Design review of the part built by this model. Coordinates are the model's own, in mm. Face numbers are marked on the shaded views. A direction names the side the tool comes from. Give positions to 0.01 mm unless a question says otherwise; leave off trailing zeros. Write each loop counter-clockwise with the first axis right and the second up, starting at its lowest first coordinate (ties: lowest second). Pieces come first, ordered by that corner, then holes. Notation, with made-up numbers: (73.5, 74) -> (101.5, 74) arc R11 cw to (101.5, 86) -> close; hole circle Ø3 at (-25, 31). An arc over 180 degrees is marked (long way). Answer as a JSON object with one key per item and string values.
Autodesk Inventor part; units mm, degrees
ref_plane "YZ Plane" through (0, 0, 0) normal (1, 0, 0) x (0, 1, 0)
ref_plane "XZ Plane" through (0, 0, 0) normal (0, 1, 0) x (-1, 0, 0)
ref_plane "XY Plane" through (0, 0, 0) normal (0, 0, 1) x (1, 0, 0)
sketch "Sketch1" plane through (0, 0, 0) normal (0, 0, 1) x (1, 0, 0)
  circle A0 centre (0, 0) radius 3.9688
  dimension "d0" = 7.9375
extrude "Extrusion1" add sketch "Sketch1" along normal blind 6.35
sketch "Sketch2" plane through (0, 0, 6.35) normal (0, 0, 1) x (1, 0, 0)
  circle A0 centre (0, 0) radius 3.9688
  circle A1 centre (0, 0) radius 2.413
  dimension "d4" = 4.826
extrude "Extrusion2" add sketch "Sketch2" along normal blind 8.89 contours A1
thread "Thread1"
sketch "Sketch3" plane through (0, 0, 15.24) normal (0, 0, 1) x (1, 0, 0)
  circle A0 centre (0, 0) radius 2.413
  circle A1 centre (0, 0) radius 1.8986
  dimension "d17" = 3.7973
extrude "Extrusion3" add sketch "Sketch3" along normal blind 18.3356 contours A1
sketch "Sketch4" plane through (0, 0, 0) normal (0, 0, -1) x (-1, 0, 0)
  circle A0 centre (0, 0) radius 3.9688
  line L0 (-2.2914, 0) -> (-1.1457, 1.9844)
  line L1 (-1.1457, 1.9844) -> (1.1457, 1.9844)
  line L2 (1.1457, 1.9844) -> (2.2914, 0)
  line L3 (2.2914, 0) -> (1.1457, -1.9844)
  line L4 (1.1457, -1.9844) -> (-1.1457, -1.9844)
  line L5 (-1.1457, -1.9844) -> (-2.2914, 0)
  dimension "d23" = 3.9688
extrude "Extrusion4" cut sketch "Sketch4" against normal blind 3.175 contours L0 L1 L2 L3 L4 L5
sketch "Sketch5" plane through (0, 0, 33.5756) normal (0, 0, 1) x (1, 0, 0)
  circle A0 centre (0, 0) radius 1.8986
  circle A1 centre (0, 0) radius 1.7526
  dimension "d32" = 3.5052
extrude "Extrusion5" add sketch "Sketch5" along normal blind 17.2244 contours A1
thread "Thread2"
chamfer "Chamfer1" distance 0.254 angle 45 3 edges at (-3.9688, 0, 0) (-3.9688, 0, 6.35) (-1.7526, 0, 50.8)
chamfer "Chamfer2" distance 0.127 angle 45 1 edges at (-2.413, 0, 15.24)
properties part number "Rod Nut Side"
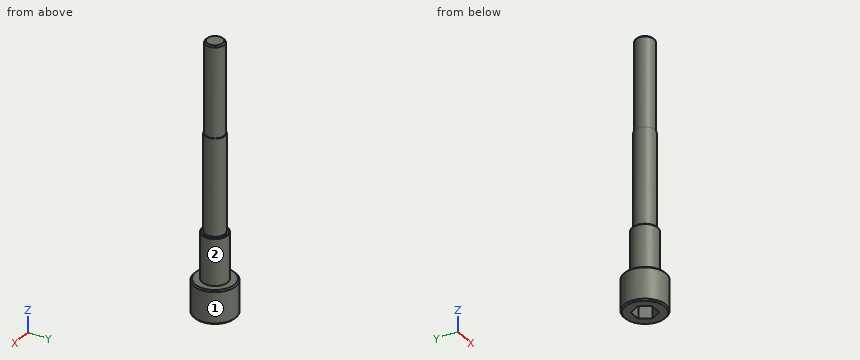
(1) We need section B-B, the plane z = 27. State the section outline as (x, y) points, then the cut area to 3 significant figures.
Here are the results:
{"outline": "circle Ø3.8 at (0, 0)", "area": "11.3 mm²"}
(2) We need section C-C, the plane z = 39. State the section outline as (x, y) points, then the cut area to 3 significant figures.
Here are the results:
{"outline": "circle Ø3.51 at (0, 0)", "area": "9.65 mm²"}
(3) Clearance check with flat-ended pins moving along their axes: pin 1 (1.5 mm diameter, centred on x = -0.5, z = 28, fed in from -Y); pin 2 (1.2 mm diameter, centred on x = -0.5, y = -1, fed in from -Z) (3 decimals); pin 3 (3 mm diameter, centred on x = 1, z = 43.5, fed in from -Y); pin 4 (4 mm diameter, centred on x = 0, y = -2, fed in from -Z). State where each tip first meets the part, or that it passes through.
Here are the results:
{"pin 1": "stops at y = -1.9", "pin 2": "stops at z = 3.175", "pin 3": "stops at y = -1.75", "pin 4": "stops at z = 0"}
(4) For line 1 along Z through (x, y) = (-1.75, -1.25); line 2 along Y through (x, z) = (-0.75, 33); line 3 along Z through (x, y) = (-1.25, -3), list the stretches that pass through material, from the lowest coordinate up.
Here are the results:
{"line 1": "z = 0 to 15.24", "line 2": "y = -1.74 to 1.74", "line 3": "z = 0 to 6.35"}
(5) For the marked faces 1 and 2, list the 3-axis set-ups (+Z, -Z, +X, -X, +Y, -Y) from which the entire face can be reached by the end or side of a thin tool; tool diameter is ignored.
Here are the results:
{"face 1": "+Z, -Z", "face 2": "+Z"}
(6) We need section A-A, the plane x = 0. State the section outline as (y, z) points (3 decimals), then the cut area to 3 significant figures.
Here are the results:
{"outline": "(-3.969, 0.254) -> (-3.715, 0) -> (-1.984, 0) -> (-1.984, 3.175) -> (1.984, 3.175) -> (1.984, 0) -> (3.715, 0) -> (3.969, 0.254) -> (3.969, 6.096) -> (3.715, 6.35) -> (2.413, 6.35) -> (2.413, 15.113) -> (2.286, 15.24) -> (1.899, 15.24) -> (1.899, 33.576) -> (1.753, 33.576) -> (1.753, 50.546) -> (1.499, 50.8) -> (-1.499, 50.8) -> (-1.753, 50.546) -> (-1.753, 33.576) -> (-1.899, 33.576) -> (-1.899, 15.24) -> (-2.286, 15.24) -> (-2.413, 15.113) -> (-2.413, 6.35) -> (-3.715, 6.35) -> (-3.969, 6.096) -> close", "area": "210 mm²"}
